Build history of the part. All positions in model axes, mm. Give positions to 0.01 mm unless a question says otherwise; leave off trailing zeros. Loops run counter-clockwise (first coordinate to the right, second up) from the corner with the lowest first, then second, coordinate; pieces in that order, holes last. Notation, with made-up numbers: (47, -23.5) -> (90, -23.5) arc R16 cw to (90, 6.5) -> close; hole circle Ø2 at (37, -1). An arc over 180 degrees is marked (long way). One line per question, with ' | ' between items. Start each with the question number.
(1) Flat gauge pins, fed straight in: pin 1 Ø10 at (x, z) = (12.5, -6.5) entering from -Y; pin 2 Ø6 at (x, y) = (27.5, 3.5) entering from +Z; pin 3 Ø19 at (x, z) = (0, 0) entering from -Y; pin 4 Ø3 at (y, z) = (0.5, -2.5) entering from +X. Where does each tip first touch, or does it go through?
(2) Slice it at B-B, the plane x = 0. Write the cut outline in (y, z).
(3) Slice it at D-D, the plane z = 0. Write the cut outline in (x, y), then the cut area to 3 significant figures.
(4) Slice it at C-C, the plane y = 0.25. Write the cut outline in (x, z).
(5) Slice it at A-A, the plane z = -62. Write the cut outline in (x, y).
(6) Drill centre lines: L1, parallel to Z at x = 34, y = 5.5; L2, parallel to Z at x = 0, y = 3.5; L3, parallel to Z at x = 4, y = -2.75. Where is each one in solid material? Low to high. Write a range as from..to.
```python
from build123d import *

# Parameters (mm, degrees)
F0_R           = 11
F1_DEPTH       = 6
F3_D           = 6
F3_DEPTH       = 18
F3_CBORE_D     = 7.5
F3_CBORE_DEPTH = 4.5
F4_D           = 4.5
F4_DEPTH       = 18
F4_CBORE_D     = 7.5
F4_CBORE_DEPTH = 4.5
F5_W           = 11
F5_H           = 1.5
F7_SIZE        = 0.5


with BuildPart() as f1:
    # F0 (on Front) → F1 (new body, symmetric)
    with BuildSketch(Plane.XZ):
        with BuildLine():
            Line((-20.738746, 12.07909), (-43.5, -27))
            Line((-43.5, -27), (-43.5, -67))
            Line((-43.5, -67), (43.5, -67))
            Line((43.5, -67), (43.5, -27))
            Line((43.5, -27), (20.738746, 12.07909))
            ThreePointArc((20.738746, 12.07909), (0, 24), (-20.738746, 12.07909))
        make_face()
        Circle(F0_R, mode=Mode.SUBTRACT)
    extrude(amount=F1_DEPTH, both=True)

    # F3
    with Locations(Plane(origin=(0, 6, 0), x_dir=(-1, 0, 0), z_dir=(0, 1, 0))):
        with Locations((-35.5, -33), (35.5, -33)):
            CounterBoreHole(F3_D / 2, F3_CBORE_D / 2, F3_CBORE_DEPTH, depth=F3_DEPTH)

    # F4
    with Locations(Plane(origin=(0, 6, 0), x_dir=(-1, 0, 0), z_dir=(0, 1, 0))):
        with Locations((-31.5, -62), (31.5, -62)):
            CounterBoreHole(F4_D / 2, F4_CBORE_D / 2, F4_CBORE_DEPTH, depth=F4_DEPTH)

    # F5 (on Top) → F6 (revolve, cut)
    with BuildSketch(Plane.XY):
        with Locations((5.5, 5.25)):
            Rectangle(F5_W, F5_H)
        Polygon((13, 4.5), (11, 4.5), (0, 4.5), (0, 3), (13, 3), align=None)
        Polygon((13, 3), (0, 3), (0, -4.5), (16, -4.5), (16, 3), align=None)
        Polygon((16, -4.5), (0, -4.5), (0, -5.5), (17, -5.5), align=None)
        Polygon((17, -5.5), (0, -5.5), (0, -6), (20, -6), (20, -5.5), align=None)
    revolve(axis=Axis((0, 3.886208, 0), (0, -1, 0)), mode=Mode.SUBTRACT)

    # F7
    f7_edges = [f1.edges().sort_by_distance(p)[0] for p in [
        (-11, 6, 0),
        (32.119373, 6, -7.460455),
        (0, 6, 24),
        (43.5, 6, -47),
        (0, 6, -67),
        (-43.5, 6, -47),
        (-32.119373, 6, -7.460455),
        (0, -6, 24),
        (32.119373, -6, -7.460455),
        (-32.119373, -6, -7.460455),
        (-43.5, -6, -47),
        (43.5, -6, -47),
        (0, -6, -67),
    ]]
    chamfer(f7_edges, length=F7_SIZE)


solid = f1.part
```
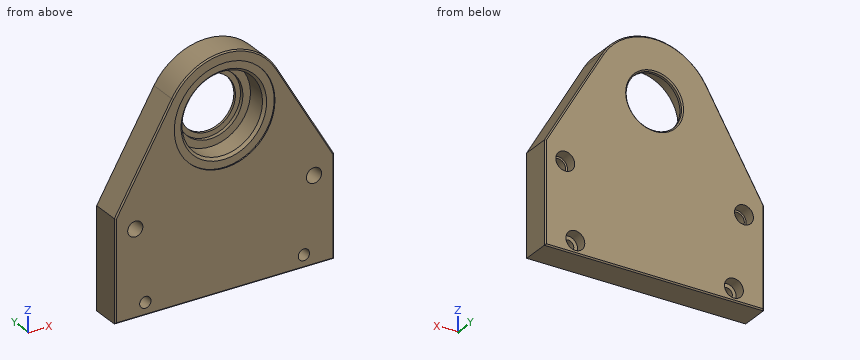
Final values:
1) pin 1: y = -5.5 | pin 2: z = 5.62 | pin 3: through | pin 4: x = 30.1
2) outline: (-6, -66.5) -> (-5.5, -67) -> (5.5, -67) -> (6, -66.5) -> (6, -11.5) -> (5.5, -11) -> (4.5, -11) -> (4.5, -13) -> (3, -13) -> (3, -16) -> (-4.5, -16) -> (-5.5, -17) -> (-5.5, -20) -> (-6, -20) -> close; (-6, 20) -> (-5.5, 20) -> (-5.5, 17) -> (-4.5, 16) -> (3, 16) -> (3, 13) -> (4.5, 13) -> (4.5, 11) -> (5.5, 11) -> (6, 11.5) -> (6, 23.5) -> (5.5, 24) -> (-5.5, 24) -> (-6, 23.5) -> close
3) outline: (-27.77, -5.5) -> (-27.2, -6) -> (-20, -6) -> (-20, -5.5) -> (-17, -5.5) -> (-16, -4.5) -> (-16, 3) -> (-13, 3) -> (-13, 4.5) -> (-11, 4.5) -> (-11, 5.5) -> (-11.5, 6) -> (-27.2, 6) -> (-27.77, 5.5) -> close; (11, 4.5) -> (13, 4.5) -> (13, 3) -> (16, 3) -> (16, -4.5) -> (17, -5.5) -> (20, -5.5) -> (20, -6) -> (27.2, -6) -> (27.77, -5.5) -> (27.77, 5.5) -> (27.2, 6) -> (11.5, 6) -> (11, 5.5) -> close | area: 301 mm2
4) outline: (-43.5, -67) -> (43.5, -67) -> (43.5, -27) -> (20.74, 12.08) arc R24 ccw to (-20.74, 12.08) -> (-43.5, -27) -> close; hole circle Ø6 at (-35.5, -33); hole circle Ø4.5 at (-31.5, -62); hole circle Ø32 at (0, 0); hole circle Ø4.5 at (31.5, -62); hole circle Ø6 at (35.5, -33)
5) outline: (-43.5, -5.5) -> (-43, -6) -> (-33.75, -6) -> (-33.75, 1.5) -> (-35.25, 1.5) -> (-35.25, 6) -> (-43, 6) -> (-43.5, 5.5) -> close; (-29.25, -6) -> (29.25, -6) -> (29.25, 1.5) -> (27.75, 1.5) -> (27.75, 6) -> (-27.75, 6) -> (-27.75, 1.5) -> (-29.25, 1.5) -> close; (33.75, -6) -> (43, -6) -> (43.5, -5.5) -> (43.5, 5.5) -> (43, 6) -> (35.25, 6) -> (35.25, 1.5) -> (33.75, 1.5) -> close
6) L1: -67..-64.8, -59.2..-36.44, -29.56..-10.69 | L2: -67..-13, 13..24 | L3: -67..-15.49, 15.49..23.66
